Autodesk Inventor part; units mm, degrees
ref_plane "Start Plane" through (0, 0, 76.231) normal (0, 0, 1) x (1, 0, 0)
ref_plane "End Plane" through (0, 0, 584.2) normal (0, 0, 1) x (1, 0, 0)
ref_plane "Work Plane4" through (-25.4, -38.131, 584.2) normal (0, 0, 1) x (1, 0, 0)
ref_plane "Start Plane" through (0, 0, 76.231) normal (0, 0, 1) x (1, 0, 0)
ref_plane "End Plane" through (0, 0, 584.2) normal (0, 0, 1) x (1, 0, 0)
sketch "Sketch" plane through (0, 0, 0) normal (0, 0, 1) x (1, 0, 0)
  line L0 (-25.4, -31.75) -> (-25.4, 31.75)
  line L1 (-19.05, 38.1) -> (19.05, 38.1)
  line L2 (25.4, 31.75) -> (25.4, -31.75)
  line L3 (19.05, -38.1) -> (-19.05, -38.1)
  arc A0 (-25.4, -31.75) -> (-19.05, -38.1) centre (-19.05, -31.75) ccw
  arc A1 (-19.05, 38.1) -> (-25.4, 31.75) centre (-19.05, 31.75) ccw
  arc A2 (25.4, 31.75) -> (19.05, 38.1) centre (19.05, 31.75) ccw
  arc A3 (19.05, -38.1) -> (25.4, -31.75) centre (19.05, -31.75) ccw
  arc A4 (-19.05, 34.925) -> (-22.225, 31.75) centre (-19.05, 31.75) ccw
  line L4 (-19.05, 34.925) -> (19.05, 34.925)
  arc A5 (22.225, 31.75) -> (19.05, 34.925) centre (19.05, 31.75) ccw
  line L5 (22.225, 31.75) -> (22.225, -31.75)
  arc A6 (19.05, -34.925) -> (22.225, -31.75) centre (19.05, -31.75) ccw
  line L6 (19.05, -34.925) -> (-19.05, -34.925)
  arc A7 (-22.225, -31.75) -> (-19.05, -34.925) centre (-19.05, -31.75) ccw
  line L7 (-22.225, -31.75) -> (-22.225, 31.75)
  line L8 (0, 55.1812) -> (0, -55.1812) construction
  line L9 (-37.4012, 0) -> (37.4012, 0) construction
  dimension "d10" = 76.2
  dimension "d11" = 50.8
  dimension "d12" = 3.175
  dimension "d15" = 38.1
  dimension "d16" = 25.4
  dimension "d17" = 6.35
extrude "Body" add sketch "Sketch" along normal up to surface (507.969 mm away) from surface at 76.231
sketch "Sketch3" plane through (0, 0, 0) normal (0, 0, 1) x (1, 0, 0)
  line L0 (0, 0) -> (10, 0)
ref_plane "Work Plane3" through (0, 0, 0) normal (0, -1, 0) x (1, 0, 0)
ref_plane "Work Plane4" through (-25.4, -38.131, 584.2) normal (0, 0, 1) x (1, 0, 0)
split "Split1" plane through (-25.4, -38.131, 584.2) removes the side toward (0, 0, 1)
ref_plane "Work Plane5" through (0, -1230.9, 76.231) normal (0, 0, -1) x (-1, 0, 0)
split "Split2" plane through (0, -1230.9, 76.231) removes the side toward (0, 0, -1)
sketch "Sketch4" plane through (0, 0, 0) normal (0, -1, 0) x (1, 0, 0)
  line L0 (-2, 76.231) -> (12, 76.231)
  line L1 (-2, 584.2) -> (12, 584.2)
  dimension "d19" = 507.969
equation "\"d10\" = G_H"
equation "\"d11\" = G_W"
equation "\"d12\" = G_T"
equation "\"d15\" = 0.5 * d10"
equation "\"d16\" = 0.5 * d11"
equation "\"d17\" = G_IR"
equation "\"G_W\" = 50.8"
equation "\"G_H\" = 76.2"
equation "\"G_T\" = 3.175"
equation "\"G_IR\" = 6.35"
equation "\"G_L\" = d19"
equation "\"G_OFFSET_START\" = -76.231"
equation "\"G_OFFSET_END\" = 0"
equation "\"d13\" = -G_OFFSET_START"
equation "\"d14\" = G_OFFSET_END + B_L"
equation "\"B_L\" = 584.2"
properties part number "AISC - 3 x 2 x 1/8 - 19.999" material "Steel, Mild"
Read the model definition and answer for the solid it produces. Units are mm, in the model's axes. A direction names the side the tool comes from. Coordinates: 2 decimals unless noted, no trailing zeros. Loops run counter-clockwise (first coordinate to the right, second up) from the corner with the lowest first, then second, coordinate; pieces in that order, holes last. Notation, with made-up numbers: (-18.5, 61.25) - (40.5, 61.25) arc R8 cw to (40.5, 68.25) - close; hole circle Ø3 at (-18, 5.5). An arc over 180 degrees is marked (long way). Answer in a Markdown table with one row per item.
1. Straight lines are drawn through the part: line 1 (Y direction, x = -7, z = 430) (3 decimals); line 2 (X direction, y = 28.5, z = 414.5) (3 decimals); line 3 (Y direction, x = -21, z = 352.5). For each, find the intervals that lie inside material, in ascending order.
Conclusion:
| item | result |
|---|---|
| line 1 | y = -38.1 to -34.925, 34.925 to 38.1 |
| line 2 | x = -25.4 to -22.225, 22.225 to 25.4 |
| line 3 | y = -37.79 to -34.26, 34.26 to 37.79 |
2. Which of the six approach directions +Z, -Z, +X, -X, +Y, -Y give full straight-line access (tool end or side, diameter ignored) to faces 4 (the face through (25.4, 0, 327)), 5 (the face through (0, 34.925, 327))?
Conclusion:
| item | result |
|---|---|
| face 4 | +Z, -Z, +X, +Y, -Y |
| face 5 | +Z, -Z |
3. Determine the mould class of faces 1 (the face through (-22.225, 0, 327)), 2 (the face through (-25.4, 0, 327)), 3 (the face through (0, 38.1, 327)) for opening direction Y: +Y half, -Y half, draft (parallel to the pull), parting line (faces both ways), or undercut.
Conclusion:
| item | result |
|---|---|
| face 1 | undercut |
| face 2 | draft |
| face 3 | +Y half |
4. Given pin 1 (12 mm diameter, centred on x = -20, z = 403.5, fed in from -Y), flat-ended and moving along its own axis, determine where the tip first touches the part or whether it passes through.
Conclusion:
| item | result |
|---|---|
| pin 1 | stops at y = -38.1 |
5. Find section A-A, the plane x = -5. Write down the section's boundary in (y, z) (3 decimals), then the cut area to 3 significant figures.
Conclusion:
| item | result |
|---|---|
| outline | (-38.1, 76.231) - (-34.925, 76.231) - (-34.925, 584.2) - (-38.1, 584.2) - close; (34.925, 76.231) - (38.1, 76.231) - (38.1, 584.2) - (34.925, 584.2) - close |
| area | 3,230 mm² |
6. Find section C-C, the plane z = 426. Write down the section's boundary in (x, y) (3 decimals), then the cut area to 3 significant figures.
Conclusion:
| item | result |
|---|---|
| outline | (-25.4, -31.75) arc R6.35 ccw to (-19.05, -38.1) - (19.05, -38.1) arc R6.35 ccw to (25.4, -31.75) - (25.4, 31.75) arc R6.35 ccw to (19.05, 38.1) - (-19.05, 38.1) arc R6.35 ccw to (-25.4, 31.75) - close; hole (-22.225, -31.75) arc R3.175 ccw to (-19.05, -34.925) - (19.05, -34.925) arc R3.175 ccw to (22.225, -31.75) - (22.225, 31.75) arc R3.175 ccw to (19.05, 34.925) - (-19.05, 34.925) arc R3.175 ccw to (-22.225, 31.75) - close |
| area | 740 mm² |
7. Find section B-B, the plane y = 16. Write down the section's boundary in (x, z) (3 decimals), then the cut area to 3 significant figures.
Conclusion:
| item | result |
|---|---|
| outline | (-25.4, 76.231) - (-22.225, 76.231) - (-22.225, 584.2) - (-25.4, 584.2) - close; (22.225, 76.231) - (25.4, 76.231) - (25.4, 584.2) - (22.225, 584.2) - close |
| area | 3,230 mm² |
